Geometry: see drawing. Coordinates: mm, zero at the bounding-box minimum. A direction names the side the tool comes from. Give positions to 0.01 mm unless a question says otherwise; leave off trailing zeros. Order: outer loops, then holes, each group sorted by start corner. A loop starts at its lowest first (then second) coordinate and runs counter-clockwise, first axis right, second up. Notation, with made-up numbers: (-8.5, 79) - (41.5, 79) arc R24 cw to (41.5, 94) - close; hole circle Ø6 at (29, 45). An arc over 180 degrees is marked (long way). Put each result on its own line as item: value. Start each with the question number.
1. First-contact query: P1, Ø2, axis at y = 13.5, z = 17, coming from the -X side; P2, Ø4, axis at x = 58, y = 45, coming from the +Z side; P3, Ø8, axis at y = 7, z = 25.5, coming from the +X side. Flat tips, straight axial feed; report the tip coordinate or a pass-through.
2. Mould query, pull axis X, two halves, no side actions, for the marked faces 3, 4 and 5. Classes: pulls with the +X half, pulls with the -X half, needs draft (parallel to the pull), parting line crosses it, or undercut.
3. Section A-A on y = 27.5. Return the cut outline in (x, z).
4. Section D-D on y = 11. Count the separate pieces of the cut face and the enclosed holes in it, plus the area to 3 significant figures.
5. Section B-B on x = 32.5. Return the cut outline in (y, z).
6. Section C-C on z = 21. Return the cut outline in (x, y).
7. Ray query, line 1 along Y through (x, z) = (58, 2); line 2 along Z through (x, y) = (59, 21); line 3 along Y through (x, z) = (31, 20.5). Return the intervals inside material, ascending. Write a range as from..to.
8. Set-up query: the marked faces 1 and 2. Return all of +Z, -Z, +X, -X, +Y, -Y with unobstructed straight access to the full face (end or side cutting, diameter ignored); none if empty.
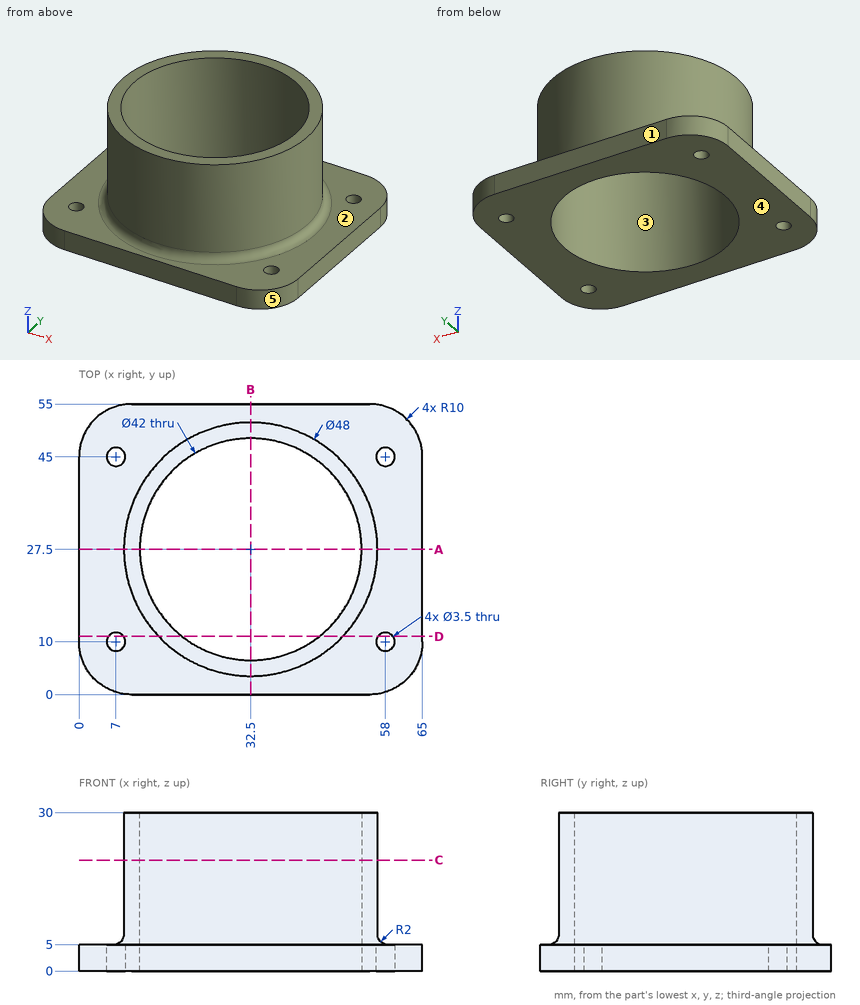
Resolved:
1. P1: x = 12.33
1. P2: z = 5
1. P3: x = 49.93
2. face 3: undercut
2. face 4: needs draft
2. face 5: pulls with the +X half
3. outline: (0, 0) - (11.5, 0) - (11.5, 30) - (8.5, 30) - (8.5, 7) arc R2 cw to (6.5, 5) - (0, 5) - close; (53.5, 0) - (65, 0) - (65, 5) - (58.5, 5) arc R2 cw to (56.5, 7) - (56.5, 30) - (53.5, 30) - close
4. separate pieces: 4
4. enclosed holes: 0
4. area: 391 mm^2
5. outline: (0, 0) - (6.5, 0) - (6.5, 30) - (3.5, 30) - (3.5, 7) arc R2 cw to (1.5, 5) - (0, 5) - close; (48.5, 0) - (55, 0) - (55, 5) - (53.5, 5) arc R2 cw to (51.5, 7) - (51.5, 30) - (48.5, 30) - close
6. outline: circle Ø48 at (32.5, 27.5); hole circle Ø42 at (32.5, 27.5)
7. line 1: 0.46..8.25, 11.75..43.25, 46.75..54.54
7. line 2: 0..5
7. line 3: 3.55..6.55, 48.45..51.45
8. face 1: +Z, -Z, +X, -X, +Y
8. face 2: +Z
